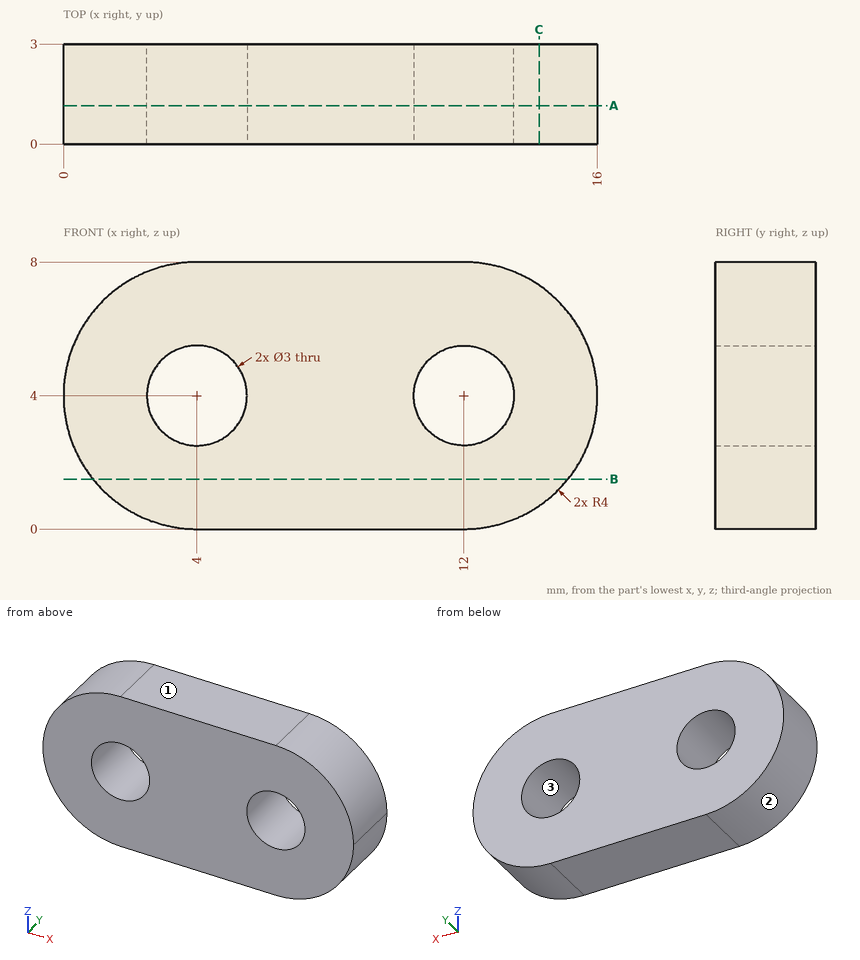
Answer from the drawing. Dimensions are ordinates in mm from the lowest x, y and z of the part. Give positions to 0.01 mm unless a question says otherwise; leave off trailing zeros. Write each loop counter-clockwise with the first axis right and the second up, starting at its lowest first coordinate (ties: lowest second). Pieces come first, ordered by that corner, then holes.
1) Given P1, Ø1.5, axis at x = 3, y = 1, coming from the -Z side; P2, Ø1.5, axis at x = 3.5, z = 4.5, coming from the -Y side, each flat-ended and moving along its own axis, determine where each tip first touches the part or whether it passes through.
2) Section A-A (y = 1.15) is taken. Write down the section's boundary in (x, z), and give its area (3 significant figures).
3) Section B-B (z = 1.5) is taken. Write down the section's boundary in (x, y).
4) For a pull along X with two mould halves and no side action, classify the marked faces 1, 2 and 3 as pulls with the +X half, pulls with the -X half, needs draft (parallel to the pull), parting line crosses it, or undercut.
5) Section C-C (x = 14.25) is taken. Write down the section's boundary in (y, z).
6) Find the intervals of material crossed by L1, parallel to Z at x = 4, y = 2.1; L2, parallel to X at y = 1.9, z = 5.25; L3, parallel to X at y = 0.5, z = 4.5, in increasing order.
Response:
1. P1: stops at z = 0.01
1. P2: passes through
2. outline: (4, 0) - (12, 0) arc R4 ccw to (12, 8) - (4, 8) arc R4 ccw to start; hole circle Ø3 at (4, 4); hole circle Ø3 at (12, 4)
2. area: 100 mm2
3. outline: (0.88, 0) - (15.12, 0) - (15.12, 3) - (0.88, 3) - close
4. face 1: needs draft
4. face 2: pulls with the -X half
4. face 3: undercut
5. outline: (0, 0.69) - (3, 0.69) - (3, 7.31) - (0, 7.31) - close
6. L1: z = 0 to 2.5, 5.5 to 8
6. L2: x = 0.2 to 3.17, 4.83 to 11.17, 12.83 to 15.8
6. L3: x = 0.03 to 2.59, 5.41 to 10.59, 13.41 to 15.97
